The listing builds one solid part. Answer for the finished solid, in the listing's coordinates (mm). A direction names the side the tool comes from. Coordinates: 2 decimals unless noted, no trailing zeros. Order: outer loops, then holes, each group sorted by start corner. A loop starts at its lowest first (then second) coordinate and runs counter-clockwise, first axis right, second up. Notation, with made-up numbers: (43.25, 75) - (66.25, 75) arc R14 ccw to (66.25, 91) - close; hole circle Ø2 at (41.25, -22). An arc over 180 degrees is marked (long way). Use one line per item in the form item = value. Start each with the question number.
Item 1: Section C-C, the plane x = -112 is taken. Write down the section's boundary in (y, z).
Item 2: Consider line 1 along Z through (x, y) = (-97, 74); line 2 along X through (y, z) = (73, -88); line 3 along X through (y, z) = (14, -43). Determine where each line is inside the solid, lowest interval first. Write a range as [from, to].
Item 3: A tool of negligible diameter and unlimited length cuts with its end or side. For faces 4 (the flat face through (2, 52, 114)), 5 (the flat face through (-164, 27, 117.5)), 6 (the flat face through (163, 27, 117.5)), from which of +Z, -Z, +X, -X, +Y, -Y can it reach the whole face along a straight path? Write none if from no direction.
Item 4: The mould has two halves that part along X. Classify faces 1 (the flat face through (-180, 67, 117.5)), 2 (the flat face through (0, 75, 130)), 3 (the flat face through (-170, 66, 128)): released by +X, released by -X, zero draft, split by the parting line, or undercut.
Item 5: Section A-A, the plane z = 98.5 is taken. Write down the section's boundary in (x, y).
Item 6: Section D-D, the plane z = -43 is taken. Write down the section's boundary in (x, y), and give its area (3 significant figures).
Item 7: Section B-B, the plane y = 36.5 is taken. Write down the section's boundary in (x, z), and give its area (3 significant figures).
Item 8: Each of these flat-tipped pins is pushed along its axis until it touches: pin 1 Ø2 at (x, z) = (71, 48.5) entering from +Y; pin 2 Ø16.5 at (x, y) = (8.5, 83) entering from +Z; pin 3 Ø16 at (y, z) = (8, -77) entering from -X; pin 4 Ø10 at (x, y) = (-182, 66.5) entering from +Z. Where does it stop, or does it pass through?
from build123d import *

# Parameters (mm, degrees)
SKETCH_1_W          = 380
SKETCH_1_H          = 275
EXTRUDE_1_DEPTH     = 90
SKETCH_2_W          = 20
SKETCH_2_H          = 20
CUT_EXTRUDE_1_DEPTH = 90
SKETCH_4_W          = 20
SKETCH_4_H          = 20
CUT_EXTRUDE_3_DEPTH = 255
SKETCH_5_W          = 20
SKETCH_5_H          = 20
CUT_EXTRUDE_4_DEPTH = 340
CUT_EXTRUDE_5_DEPTH = 77
SKETCH_7_W          = 60
SKETCH_7_H          = 15
CUT_EXTRUDE_6_DEPTH = 15
CUT_EXTRUDE_7_DEPTH = 20
CUT_EXTRUDE_8_DEPTH = 20
CUT_EXTRUDE_9_DEPTH = 20


with BuildPart() as part:
    # 草圖1 → 填料-伸長1 (new body)
    with BuildSketch(Plane(origin=(0, 0, 0), x_dir=(1, 0, 0), z_dir=(0, 1, 0))):
        Rectangle(SKETCH_1_W, SKETCH_1_H)
    extrude(amount=EXTRUDE_1_DEPTH)

    # 草圖2 → 除料-伸長1 (cut)
    with BuildSketch(Plane(origin=(0, 90, 0), x_dir=(1, 0, 0), z_dir=(0, 1, 0))):
        with Locations((-180, -127.5)):
            Rectangle(SKETCH_2_W, SKETCH_2_H)
        with Locations((180, -127.5)):
            Rectangle(SKETCH_2_W, SKETCH_2_H)
    extrude(amount=-CUT_EXTRUDE_1_DEPTH, mode=Mode.SUBTRACT)

    # 草圖4 → 除料-伸長3 (cut)
    with BuildSketch(Plane.XY.offset(117.5)):
        with Locations((-180, 10)):
            Rectangle(SKETCH_4_W, SKETCH_4_H)
        with Locations((180, 10)):
            Rectangle(SKETCH_4_W, SKETCH_4_H)
    extrude(amount=-CUT_EXTRUDE_3_DEPTH, mode=Mode.SUBTRACT)

    # 草圖5 → 除料-伸長4 (cut)
    with BuildSketch(Plane.ZY.offset(170)):
        with Locations((127.5, 10)):
            Rectangle(SKETCH_5_W, SKETCH_5_H)
    extrude(amount=-CUT_EXTRUDE_4_DEPTH, mode=Mode.SUBTRACT)

    # 草圖6 → 除料-伸長5 (cut)
    with BuildSketch(Plane(origin=(0, 90, 0), x_dir=(1, 0, 0), z_dir=(0, 1, 0))):
        Polygon((-166.5, 134), (166.5, 134), (166.5, -90.5), (143, -114), (-143, -114), (-166.5, -90.5), align=None)
    extrude(amount=-CUT_EXTRUDE_5_DEPTH, mode=Mode.SUBTRACT)

    # 草圖7 → 除料-伸長6 (cut)
    with BuildSketch(Plane.XY.offset(137.5)):
        with Locations((0, 82.5)):
            Rectangle(SKETCH_7_W, SKETCH_7_H)
    extrude(amount=-CUT_EXTRUDE_6_DEPTH, mode=Mode.SUBTRACT)

    # 草圖9 → 除料-伸長7 (cut)
    with BuildSketch(Plane.XY.offset(137.5)):
        Polygon((-170, 20), (-170, 43.5), (-146.5, 20), align=None)
        Polygon((170, 43.5), (146.5, 20), (170, 20), align=None)
    extrude(amount=-CUT_EXTRUDE_7_DEPTH, mode=Mode.SUBTRACT)

    # 草圖10 → 除料-伸長8 (cut)
    with BuildSketch(Plane(origin=(190, 0, 0), x_dir=(0, 0, -1), z_dir=(1, 0, 0))):
        Polygon((-94, 20), (-117.5, 20), (-117.5, 43.5), align=None)
    cut_extrude_8 = extrude(amount=-CUT_EXTRUDE_8_DEPTH, mode=Mode.SUBTRACT)

    # 鏡射1: 除料-伸長8 across plane
    add(cut_extrude_8.mirror(Plane(origin=(0, 0, 0), x_dir=(0, 0, 1), z_dir=(1, 0, 0))), mode=Mode.SUBTRACT)

    # 草圖11 → 除料-伸長9 (cut)
    with BuildSketch(Plane.XZ):
        Polygon((-146.5, 117.5), (-170, 117.5), (-170, 94), align=None)
        Polygon((170, 94), (146.5, 117.5), (170, 117.5), align=None)
    extrude(amount=-CUT_EXTRUDE_9_DEPTH, mode=Mode.SUBTRACT)


solid = part.part
Response:
q1.outline = (0, -137.5) - (90, -137.5) - (90, -134) - (13, -134) - (13, 114) - (90, 114) - (90, 137.5) - (20, 137.5) - (20, 117.5) - (0, 117.5) - close
q2.line_1 = [-137.5, -134], [114, 137.5]
q2.line_2 = [-190, -166.5], [166.5, 190]
q2.line_3 = [-170, -166.5], [166.5, 170]
q3.face_4 = +Y
q3.face_5 = +Z, -X, -Y
q3.face_6 = +Z, +X, -Y
q4.face_1 = zero draft
q4.face_2 = undercut
q4.face_3 = released by -X
q5.outline = (-190, 24.5) - (-170, 24.5) - (-170, 20) - (-165.5, 20) - (-165.5, 0) - (165.5, 0) - (165.5, 20) - (170, 20) - (170, 24.5) - (190, 24.5) - (190, 90) - (158.5, 90) - (158.5, 13) - (-158.5, 13) - (-158.5, 90) - (-190, 90) - close
q6.outline = (-190, 20) - (-170, 20) - (-170, 0) - (170, 0) - (170, 20) - (190, 20) - (190, 90) - (166.5, 90) - (166.5, 13) - (-166.5, 13) - (-166.5, 90) - (-190, 90) - close
q6.area = 7,760 mm2
q7.outline = (-190, -137.5) - (190, -137.5) - (190, 110.5) - (170, 110.5) - (170, 117.5) - (163, 117.5) - (163, 137.5) - (-163, 137.5) - (-163, 117.5) - (-170, 117.5) - (-170, 110.5) - (-190, 110.5) - close; hole (-166.5, -134) - (166.5, -134) - (166.5, 90.5) - (143, 114) - (-143, 114) - (-166.5, 90.5) - close
q7.area = 21,100 mm2
q8.pin_1 = 13
q8.pin_2 = 137.5
q8.pin_3 = -170
q8.pin_4 = 117.5
